The drawing under review shows one solid part. Ordinate dimensions are in mm from its lowest x, y, z. A direction names the side the tool comes from. Coordinates: 2 decimals unless noted, no trailing zeros. Write each loop counter-clockwise with the first axis right and the second up, starting at its lowest first coordinate (ties: lowest second). Pieces come first, ordered by that corner, then holes.
Q1. Machinability: for the marked faces 1, 2 and 3, which of the approach directions +Z, -Z, +X, -X, +Y, -Y give a long, thin tool a straight path to every point of the face, cutting with its end or side? Answer none if there is none.
Q2. Insertion check: pin 1 (2 mm diameter, centred on y = 62.5, z = 70, fed in from +X); pin 2 (1 mm diameter, centred on y = 51.5, z = 14, fed in from -X); pin 3 (10 mm diameter, centred on x = 70.5, y = 47, fed in from +Z); pin 4 (1 mm diameter, centred on x = 71, y = 38, fed in from -Z). Each pin has a flat end and moves straight along its axis. Give the tip position at first contact, or say it passes through.
Q3. For probe 1 along X at (y, z) = (34.5, 13); probe 2 along X at (y, z) = (32.5, 93.5); probe 3 along Z at (x, y) = (87.5, 61.5), list the stretches that pass through material, from the lowest coordinate up.
Q4. Take a section at B-B (z = 11.5). Give the boundary of the cut face in (x, y).
Q5. Take a section at C-C (x = 94.5). Give the boundary of the cut face in (y, z), and give its area (3 significant figures).
Q6. Take a section at A-A (y = 54). Give the boundary of the cut face in (x, z).
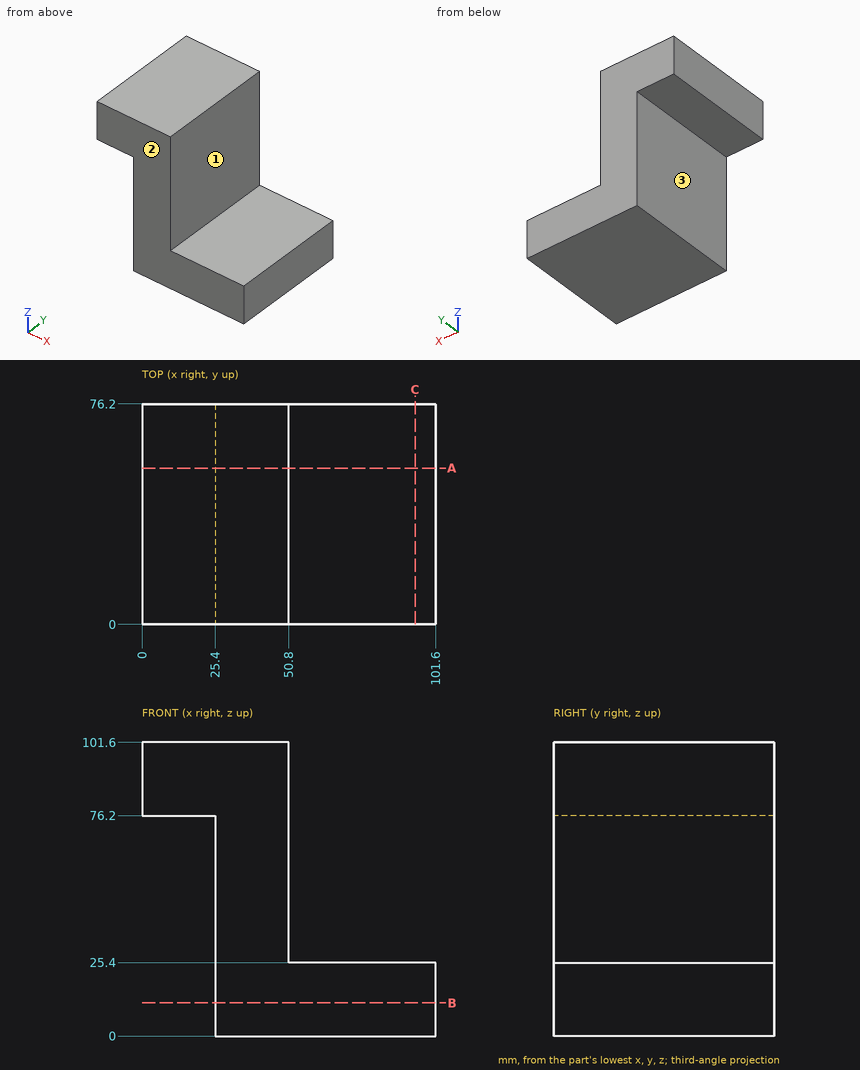
Response:
1. face 1: +Z, +X, +Y, -Y
1. face 2: +Z, -Z, +X, -X, -Y
1. face 3: -Z, -X, +Y, -Y
2. pin 1: stops at x = 50.8
2. pin 2: stops at x = 25.4
2. pin 3: stops at z = 25.4
2. pin 4: stops at z = 0
3. probe 1: x = 25.4 to 101.6
3. probe 2: x = 0 to 50.8
3. probe 3: z = 0 to 25.4
4. outline: (25.4, 0) - (101.6, 0) - (101.6, 76.2) - (25.4, 76.2) - close
5. outline: (0, 0) - (76.2, 0) - (76.2, 25.4) - (0, 25.4) - close
5. area: 1,940 mm2
6. outline: (0, 76.2) - (25.4, 76.2) - (25.4, 0) - (101.6, 0) - (101.6, 25.4) - (50.8, 25.4) - (50.8, 101.6) - (0, 101.6) - close
